```python
from build123d import *

# Parameters (mm, degrees)
F1_DEPTH = 25.4
F3_DEPTH = 12.7


with BuildPart() as f1:
    # F0 (on Front) → F1 (new body)
    with BuildSketch(Plane.XZ):
        Polygon((0, 31.75), (0, 0), (38.1, 0), (38.1, 31.75), (25.4, 31.75), (25.4, 25.4), (12.7, 25.4), (12.7, 31.75), align=None)
    extrude(amount=F1_DEPTH)

    # F2 (on face) → F3 (cut)
    with BuildSketch(Plane.XZ.offset(25.4)):
        Polygon((0, 31.75), (0, 10.059285), (38.1, 10.059285), (38.1, 31.75), (25.4, 31.75), (25.4, 25.4), (12.7, 25.4), (12.7, 31.75), align=None)
    extrude(amount=-F3_DEPTH, mode=Mode.SUBTRACT)


solid = f1.part
```
Design review of the part built by this model. Coordinates are the model's own, in mm. A direction names the side the tool comes from. Give positions to 0.01 mm unless a question says otherwise; leave off trailing zeros. Write each loop counter-clockwise with the first axis right and the second up, starting at its lowest first coordinate (ties: lowest second). Pieces come first, ordered by that corner, then holes.
(1) Add section C-C (y = -6.75). Give the boundary of the cut face in (x, z), and give its area (3 significant figures).
Checked values:
outline: (0, 0) - (38.1, 0) - (38.1, 31.75) - (25.4, 31.75) - (25.4, 25.4) - (12.7, 25.4) - (12.7, 31.75) - (0, 31.75) - close
area: 1,130 mm2
(2) Add section B-B (x = 27.5). Give the boundary of the cut face in (y, z).
Checked values:
outline: (-25.4, 0) - (0, 0) - (0, 31.75) - (-12.7, 31.75) - (-12.7, 10.06) - (-25.4, 10.06) - close
(3) Wall thickness on line 1 along X through (y, z) = (-7, 27); line 2 along Y through (x, z) = (35.5, 11); line 3 along Z through (x, y) = (25, -3.5): over which ranges is each line inside the solid? List them lowest first.
Checked values:
line 1: x = 0 to 12.7, 25.4 to 38.1
line 2: y = -12.7 to 0
line 3: z = 0 to 25.4
(4) Add section D-D (z = 21.5). Give the boundary of the cut face in (x, y).
Checked values:
outline: (0, -12.7) - (38.1, -12.7) - (38.1, 0) - (0, 0) - close
(5) Tool access review of faces 4 (the face through (19, -13, 0)), 5 (the face through (19, -12.7, 21)), 6 (the face through (12.7, -6, 29)): name each direction out of +Z, -Z, +X, -X, +Y, -Y from which nothing blocks a thin tool from reaching the whole face with its end or side.
Checked values:
face 4: -Z, +X, -X, +Y, -Y
face 5: +Z, +X, -X, -Y
face 6: +Z, +Y, -Y
(6) Clearance check with flat-ended pins moving along their axes: pin 1 Ø6.5 at (x, z) = (16.5, 23) entering from -Y; pin 2 Ø10 at (x, y) = (10.5, -18.5) entering from +Z; pin 3 Ø1.5 at (x, y) = (19, -10) entering from +Z. State where each tip first meets the part, or that it passes through.
Checked values:
pin 1: stops at y = -12.7
pin 2: stops at z = 10.06
pin 3: stops at z = 25.4
(7) Mouldability with a two-part tool opening along X and no side actions: class faces 1 (the face through (0, -10, 13)), 2 (the face through (32, -6, 31.75)), 3 (the face through (19, -6, 25.4)) as +X half, -X half, draft (parallel to the pull), parting line (faces both ways), or undercut.
Checked values:
face 1: -X half
face 2: draft
face 3: undercut
(8) Add section A-A (z = 27). Give the boundary of the cut face in (x, y).
Checked values:
outline: (0, -12.7) - (12.7, -12.7) - (12.7, 0) - (0, 0) - close; (25.4, -12.7) - (38.1, -12.7) - (38.1, 0) - (25.4, 0) - close
